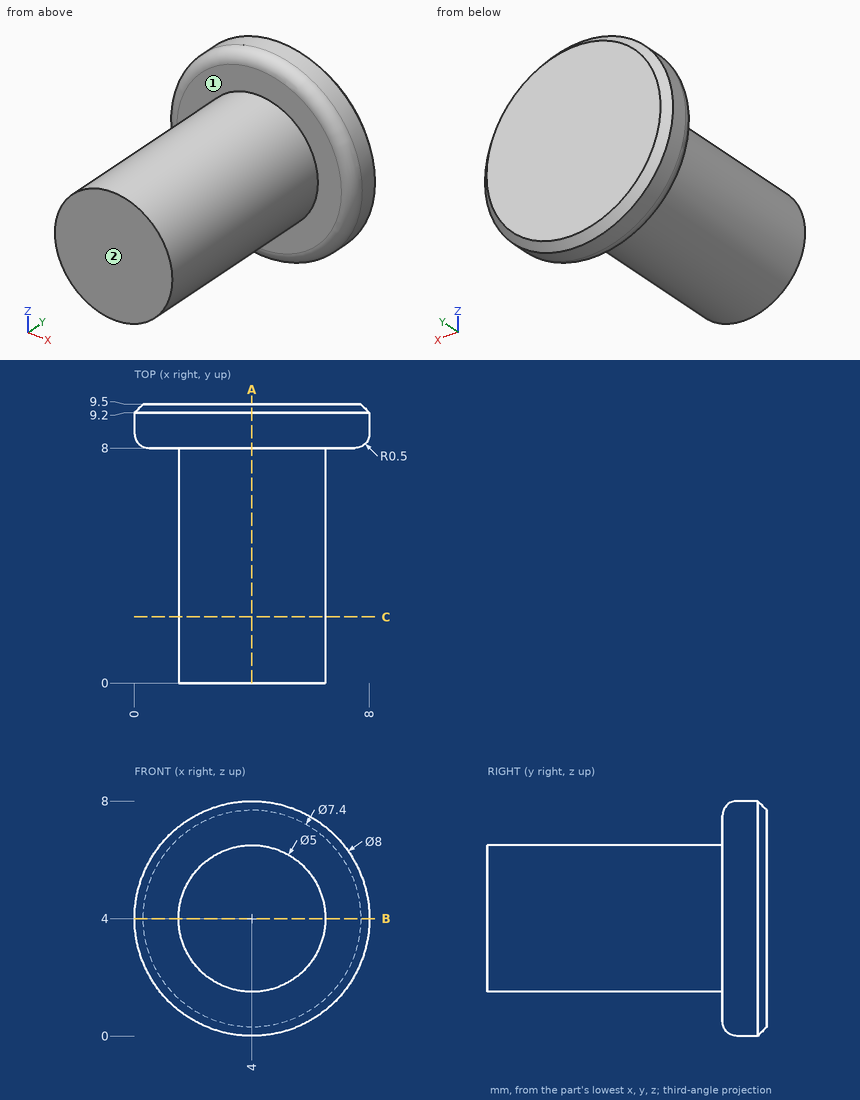
Study the drawing (mm; zero at the part's minimum x, y, z) and answer. A direction names the side the tool comes from. Give positions to 0.01 mm unless a question says otherwise; leave off trailing zeros. Order: outer loops, then holes, each group sorted by start corner. A loop starts at its lowest first (then second) coordinate and runs counter-clockwise, first axis right, second up. Notation, with made-up numbers: (-19.5, 45.25) - (18.5, 45.25) arc R31 cw to (18.5, 74.25) - close; hole circle Ø9 at (56, 35.25). An arc over 180 degrees is marked (long way). Answer in a Markdown table with one row per item. Add a question column.
Q1. Find the intervals of material crossed by line 1 along Y through (x, z) = (3.5, 7.25); line 2 along X through (y, z) = (8.75, 3.75); line 3 along Z through (x, y) = (2.25, 5.25), in increasing order. Write a range as [from, to].
Q2. The part is cut by section B-B (z = 4). Determine the outline of the cut face in (x, y).
Q3. Which of the six approach directions +Z, -Z, +X, -X, +Y, -Y give full straight-line access (tool end or side, diameter ignored) to the marked faces 1 and 2?
Q4. The part is cut by section C-C (y = 2.25). Determine the outline of the cut face in (x, z), then the cut area to 3 significant figures.
Q5. The part is cut by section A-A (x = 4). Determine the outline of the cut face in (y, z), then the cut area to 3 significant figures.
Q6. Given P1, Ø1.5, axis at y = 1.5, z = 4.5, coming from the -X side; P2, Ø1, axis at y = 5.5, z = 6.5, coming from the +X side, each flat-ended and moving along its own axis, determine where each tip first touches the part or whether it passes through.
Determined:
| question | item | result |
|---|---|---|
| 1 | line 1 | y = [8, 9.5] |
| 1 | line 2 | x = [0.01, 7.99] |
| 1 | line 3 | z = [2.21, 5.79] |
| 2 | outline | (0, 8.5) arc R0.5 ccw to (0.5, 8) - (1.5, 8) - (1.5, 0) - (6.5, 0) - (6.5, 8) - (7.5, 8) arc R0.5 ccw to (8, 8.5) - (8, 9.2) - (7.7, 9.5) - (0.3, 9.5) - (0, 9.2) - close |
| 3 | face 1 | -Y |
| 3 | face 2 | +Z, -Z, +X, -X, -Y |
| 4 | outline | circle Ø5 at (4, 4) |
| 4 | area | 19.6 mm² |
| 5 | outline | (0, 1.5) - (8, 1.5) - (8, 0.5) arc R0.5 ccw to (8.5, 0) - (9.2, 0) - (9.5, 0.3) - (9.5, 7.7) - (9.2, 8) - (8.5, 8) arc R0.5 ccw to (8, 7.5) - (8, 6.5) - (0, 6.5) - close |
| 5 | area | 51.8 mm² |
| 6 | P1 | stops at x = 1.5 |
| 6 | P2 | stops at x = 5.5 |
